```python
from build123d import *

# Parameters (mm, degrees)
SPROKET_DEPTH       = 9
SKETCH3_R           = 12.5
CUT_EXTRUDE1_DEPTH  = 7
SKETCH4_R           = 4.5
BOSS_EXTRUDE1_DEPTH = 7


with BuildPart() as part:
    # Sprocket → Sproket (new body)
    with BuildSketch(Plane(origin=(-521.333895642, -864.335014518, -1401.843992528), x_dir=(1, 0, 0), z_dir=(0, 0, 1))):
        with BuildLine():
            ThreePointArc((502.621153074, 859.818847383), (503.02864119, 858.378492088), (503.546815178, 856.974153932))
            ThreePointArc((503.546815178, 856.974153932), (503.819037022, 856.702761655), (504.203425444, 856.704771932))
            ThreePointArc((504.203425444, 856.704771932), (509.005673001, 855.369858884), (508.795597259, 850.389955006))
            ThreePointArc((508.795597259, 850.389955006), (508.675219652, 850.024896474), (508.849505331, 849.682284445))
            ThreePointArc((508.849505331, 849.682284445), (510.025789743, 848.756528039), (511.270450563, 847.924969632))
            ThreePointArc((511.270450563, 847.924969632), (511.650203039, 847.865416653), (511.959998194, 848.092980848))
            ThreePointArc((511.959998194, 848.092980848), (516.629740281, 849.835703798), (519.386899492, 845.683397507))
            ThreePointArc((519.386899492, 845.683397507), (519.504087984, 845.317302769), (519.846470359, 845.142566367))
            ThreePointArc((519.846470359, 845.142566367), (521.342250401, 845.085016331), (522.837979924, 845.143864722))
            ThreePointArc((522.837979924, 845.143864722), (523.180210493, 845.318898255), (523.297081161, 845.685094579))
            ThreePointArc((523.297081161, 845.685094579), (526.05063502, 849.839792593), (530.721888079, 848.101123761))
            ThreePointArc((530.721888079, 848.101123761), (531.031880649, 847.873828563), (531.411581288, 847.933711155))
            ThreePointArc((531.411581288, 847.933711155), (532.655519825, 848.766349647), (533.831000211, 849.693126751))
            ThreePointArc((533.831000211, 849.693126751), (534.004988429, 850.035889936), (533.884293987, 850.400843839))
            ThreePointArc((533.884293987, 850.400843839), (533.669895633, 855.380563489), (538.470982641, 856.719644514))
            ThreePointArc((538.470982641, 856.719644514), (538.855372663, 856.717967897), (539.127358829, 856.989596368))
            ThreePointArc((539.127358829, 856.989596368), (539.644313618, 858.394383784), (540.050551314, 859.835092247))
            ThreePointArc((540.050551314, 859.835092247), (539.989839594, 860.214661197), (539.677681217, 860.438972694))
            ThreePointArc((539.677681217, 860.438972694), (536.577223534, 864.341630328), (539.674292437, 868.246977772))
            ThreePointArc((539.674292437, 868.246977772), (539.986255988, 868.471560146), (540.046638209, 868.851181652))
            ThreePointArc((540.046638209, 868.851181652), (539.639150093, 870.291536947), (539.120976106, 871.695875104))
            ThreePointArc((539.120976106, 871.695875104), (538.848754261, 871.967267381), (538.464365839, 871.965257104))
            ThreePointArc((538.464365839, 871.965257104), (533.662118282, 873.300170152), (533.872194024, 878.280074029))
            ThreePointArc((533.872194024, 878.280074029), (533.992571631, 878.645132562), (533.818285952, 878.98774459))
            ThreePointArc((533.818285952, 878.98774459), (532.642001541, 879.913500997), (531.39734072, 880.745059403))
            ThreePointArc((531.39734072, 880.745059403), (531.017588244, 880.804612382), (530.70779309, 880.577048188))
            ThreePointArc((530.70779309, 880.577048188), (526.038051002, 878.834325238), (523.280891791, 882.986631528))
            ThreePointArc((523.280891791, 882.986631528), (523.163703299, 883.352726267), (522.821320924, 883.527462669))
            ThreePointArc((522.821320924, 883.527462669), (521.325540883, 883.585012705), (519.829811359, 883.526164313))
            ThreePointArc((519.829811359, 883.526164313), (519.48758079, 883.35113078), (519.370710122, 882.984934457))
            ThreePointArc((519.370710122, 882.984934457), (516.617156263, 878.830236442), (511.945903204, 880.568905275))
            ThreePointArc((511.945903204, 880.568905275), (511.635910634, 880.796200472), (511.256209995, 880.736317881))
            ThreePointArc((511.256209995, 880.736317881), (510.012271459, 879.903679389), (508.836791072, 878.976902284))
            ThreePointArc((508.836791072, 878.976902284), (508.662802855, 878.6341391), (508.783497297, 878.269185196))
            ThreePointArc((508.783497297, 878.269185196), (508.99789565, 873.289465546), (504.196808642, 871.950384521))
            ThreePointArc((504.196808642, 871.950384521), (503.81241862, 871.952061138), (503.540432454, 871.680432668))
            ThreePointArc((503.540432454, 871.680432668), (503.023477665, 870.275645251), (502.617239969, 868.834936788))
            ThreePointArc((502.617239969, 868.834936788), (502.677951689, 868.455367839), (502.990110067, 868.231056341))
            ThreePointArc((502.990110067, 868.231056341), (506.090567749, 864.328398708), (502.993498846, 860.423051264))
            ThreePointArc((502.993498846, 860.423051264), (502.681535295, 860.198468889), (502.621153074, 859.818847383))
        make_face()
    sproket = extrude(amount=SPROKET_DEPTH)

    # Sketch3 → Cut-Extrude1 (cut)
    with BuildSketch(Plane.XY.offset(-1392.843992528)):
        Circle(SKETCH3_R)
    cut_extrude1 = extrude(amount=-CUT_EXTRUDE1_DEPTH, mode=Mode.SUBTRACT)

    # Mirror1: Sproket, Cut-Extrude1 across plane
    add(sproket.mirror(Plane(origin=(9.113348653, 2.199432046, -1401.843992528), x_dir=(1, 0, 0), z_dir=(0, 0, 1))))
    add(cut_extrude1.mirror(Plane(origin=(9.113348653, 2.199432046, -1401.843992528), x_dir=(1, 0, 0), z_dir=(0, 0, 1))), mode=Mode.SUBTRACT)

    # Sketch4 → Boss-Extrude1 (add)
    with BuildSketch(Plane(origin=(0, 0, -1403.843992528), x_dir=(-1, 0, 0), z_dir=(0, 0, -1))):
        Circle(SKETCH4_R)
        with BuildLine():
            Line((-1.303840481, 1.45), (1.303840481, 1.45))
            ThreePointArc((1.303840481, 1.45), (0, -1.95), (-1.303840481, 1.45))
        make_face(mode=Mode.SUBTRACT)
    extrude(amount=BOSS_EXTRUDE1_DEPTH)


solid = part.part
```
Here's how the part is built. I have some questions about the finished solid (model axes, mm). A direction names the side the tool comes from. Give positions to 0.01 mm unless a question says otherwise; leave off trailing zeros. Order: outer loops, then holes, each group sorted by start corner. A loop starts at its lowest first (then second) coordinate and runs counter-clockwise, first axis right, second up. Notation, with made-up numbers: M 64.5,52.5 L 82.5,52.5 A16 ccw 82.5,61.5 Z; hole C 46.25,70.5 d4. An arc over 180 degrees is marked long. Use a Markdown table: item, result. Add a question column.
1. Suppose I cut it at D-D (y = 0). List the corners of the cut face in (x, z) for me, and give its area (3 significant figures).
2. If we mould it in two halves opening along X, with no side actions, what happens to faces 1 (the cylindrical face through (11.305, -15.581, -1401.718)), 2 (the cylindrical face through (-0.01, -19.25, -1401.72)), 3 (the flat face through (0, -5, -1403.844))? For each: +X half, -X half, draft (parallel to the pull), parting line (faces both ways), or undercut.
3. Suppose I cut it at B-B (x = 0). List the corners of the cut face in (y, z) for me, and give its area (3 significant figures).
4. On a 3-axis mill with a long thin cutter (end or side, diameter ignored), from which of +Z, -Z, +X, -X, +Y, -Y can I reach the whole of each face in a straight line? I mean faces 4 (the cylindrical face through (11.923, 3.755, -1407.393)), 5 (the cylindrical face through (-12.29, 9.02, -1401.72)). Say none if no direction works.
5. Suppose I cut it at A-A (x = -16). List the corners of the cut face in (y, z) for me, and give its area (3 significant figures).
6. Suppose I cut it at C-C (z = -1404.5). Give the number of separate pieces and of enclosed holes in the cut face, and give its area (3 significant figures).
7. For pin 1 Ø20 at (x, y) = (0, 0) entering from +Z; pin 2 Ø1 at (y, z) = (9, -1407.5) entering from -X; pin 3 Ø6 at (y, z) = (8.5, -1395.5) entering from -X, each with a flat end and sliding along its axis, tell me the tip position at first contact or that it passes through.
8. I need wall thicknesses on probe 1 along X at (y, z) = (2.5, -1407.5); probe 2 along Z at (x, y) = (-6, 4); probe 3 along Y at (x, z) = (0, -1395.25). Which ranges of each line are inside material? Lowest first, please. Write a range as from..to.
Results list:
| question | item | result |
|---|---|---|
| 1 | outline | M -15.24,-1410.84 L -12.5,-1410.84 L -12.5,-1403.84 L -4.5,-1403.84 L -4.5,-1410.84 L -1.95,-1410.84 L -1.95,-1403.84 L 1.95,-1403.84 L 1.95,-1410.84 L 4.5,-1410.84 L 4.5,-1403.84 L 12.5,-1403.84 L 12.5,-1410.84 L 15.24,-1410.84 L 15.24,-1392.84 L 12.5,-1392.84 L 12.5,-1399.84 L -12.5,-1399.84 L -12.5,-1392.84 L -15.24,-1392.84 Z |
| 1 | area | 234 mm² |
| 2 | face 1 | +X half |
| 2 | face 2 | parting line |
| 2 | face 3 | undercut |
| 3 | outline | M -19.25,-1410.84 L -12.5,-1410.84 L -12.5,-1403.84 L -4.5,-1403.84 L -4.5,-1410.84 L -1.95,-1410.84 L -1.95,-1403.84 L 1.45,-1403.84 L 1.45,-1410.84 L 4.5,-1410.84 L 4.5,-1403.84 L 12.5,-1403.84 L 12.5,-1410.84 L 19.25,-1410.84 L 19.25,-1392.84 L 12.5,-1392.84 L 12.5,-1399.84 L -12.5,-1399.84 L -12.5,-1392.84 L -19.25,-1392.84 Z |
| 3 | area | 382 mm² |
| 4 | face 4 | -Z |
| 4 | face 5 | +Z, -Z |
| 5 | outline | M -7.34,-1410.84 L -2.35,-1410.84 L -2.35,-1392.84 L -7.34,-1392.84 Z; M 2.34,-1410.84 L 7.32,-1410.84 L 7.32,-1392.84 L 2.34,-1392.84 Z |
| 5 | area | 179 mm² |
| 6 | separate pieces | 2 |
| 6 | enclosed holes | 2 |
| 6 | area | 484 mm² |
| 7 | pin 1 | stops at z = -1399.84 |
| 7 | pin 2 | stops at x = -12.72 |
| 7 | pin 3 | stops at x = -18.45 |
| 8 | probe 1 | x = -16.13..-12.25, -3.74..3.74, 12.25..16.11 |
| 8 | probe 2 | z = -1403.84..-1399.84 |
| 8 | probe 3 | y = -19.25..-12.5, 12.5..19.25 |
